from build123d import *

# Parameters (mm, degrees)
EXTRUDE_3_DEPTH = 1.169927
EXTRUDE_4_DEPTH = 5
EXTRUDE_5_DEPTH = 5


with BuildPart() as part:
    # 草图2 → 凸台-拉伸3 (new body)
    with BuildSketch(Plane(origin=(0, 15, 0), x_dir=(1, 0, 0), z_dir=(0, 1, 0))):
        with BuildLine():
            Line((-24.853345035, 10.461479878), (-24.853345035, 0.41148))
            Line((-24.853345035, 0.41148), (-2.753344966, 0.41148))
            Line((-2.753344966, 0.41148), (-2.753344966, 10.461479878))
            Line((-2.753344966, 10.461479878), (0.013999939, 10.461479878))
            ThreePointArc((0.013999939, 10.461479878), (3.195980454, 9.143460393), (4.513999939, 5.961479878))
            Line((4.513999939, 5.961479878), (4.513999939, -14.938520122))
            ThreePointArc((4.513999939, -14.938520122), (3.195980454, -18.120500638), (0.013999939, -19.438520122))
            Line((0.013999939, -19.438520122), (-27.986000061, -19.438520122))
            ThreePointArc((-27.986000061, -19.438520122), (-31.167980576, -18.120500638), (-32.486000061, -14.938520122))
            Line((-32.486000061, -14.938520122), (-32.486000061, 5.961479878))
            ThreePointArc((-32.486000061, 5.961479878), (-31.167980576, 9.143460393), (-27.986000061, 10.461479878))
            Line((-27.986000061, 10.461479878), (-24.853345035, 10.461479878))
        make_face()
    extrude(amount=EXTRUDE_3_DEPTH)

    # 草图4 → 凸台-拉伸4 (add)
    with BuildSketch(Plane.XZ.offset(-15)):
        with BuildLine():
            Line((-23.193000031, 0.4), (-28.386000061, 0.4))
            Line((-28.386000061, 0.4), (-28.386000061, -0.81148))
            Line((-28.386000061, -0.81148), (-24.853345035, -0.81148))
            Line((-24.853345035, -0.81148), (-24.853345035, -10.461479878))
            Line((-24.853345035, -10.461479878), (-27.986000061, -10.461479878))
            ThreePointArc((-27.986000061, -10.461479878), (-31.167980576, -9.143460393), (-32.486000061, -5.961479878))
            Line((-32.486000061, -5.961479878), (-32.486000061, 14.938520122))
            ThreePointArc((-32.486000061, 14.938520122), (-31.167980576, 18.120500638), (-27.986000061, 19.438520122))
            Line((-27.986000061, 19.438520122), (0.013999939, 19.438520122))
            ThreePointArc((0.013999939, 19.438520122), (3.195980454, 18.120500638), (4.513999939, 14.938520122))
            Line((4.513999939, 14.938520122), (4.513999939, -5.961479878))
            ThreePointArc((4.513999939, -5.961479878), (3.195980454, -9.143460393), (0.013999939, -10.461479878))
            Line((0.013999939, -10.461479878), (-2.753344966, -10.461479878))
            Line((-2.753344966, -10.461479878), (-2.753344966, -0.81148))
            Line((-2.753344966, -0.81148), (0.4, -0.81148))
            Line((0.4, -0.81148), (0.4, 0.4))
            Line((0.4, 0.4), (-5.193000031, 0.4))
            Line((-5.193000031, 0.4), (-5.193000031, 3.4))
            Line((-5.193000031, 3.4), (-23.193000031, 3.4))
            Line((-23.193000031, 3.4), (-23.193000031, 0.4))
        make_face()
    extrude(amount=EXTRUDE_4_DEPTH)

    # 草图5 → 凸台-拉伸5 (add)
    with BuildSketch(Plane.XZ.offset(-10)):
        with BuildLine():
            Line((-2.753344966, -8.561479878), (0.013999939, -8.561479878))
            ThreePointArc((0.013999939, -8.561479878), (1.85247757, -7.799957509), (2.613999939, -5.961479878))
            Line((2.613999939, -5.961479878), (2.613999939, 14.938520122))
            ThreePointArc((2.613999939, 14.938520122), (1.85247757, 16.776997753), (0.013999939, 17.538520122))
            Line((0.013999939, 17.538520122), (-27.986000061, 17.538520122))
            ThreePointArc((-27.986000061, 17.538520122), (-29.824477692, 16.776997753), (-30.586000061, 14.938520122))
            Line((-30.586000061, 14.938520122), (-30.586000061, -5.961479878))
            ThreePointArc((-30.586000061, -5.961479878), (-29.824477692, -7.799957509), (-27.986000061, -8.561479878))
            Line((-27.986000061, -8.561479878), (-24.768224203, -8.561479878))
            Line((-24.768224203, -8.561479878), (-24.768224203, -7.061479878))
            Line((-24.768224203, -7.061479878), (-27.986000061, -7.061479878))
            ThreePointArc((-27.986000061, -7.061479878), (-28.76381752, -6.739297337), (-29.086000061, -5.961479878))
            Line((-29.086000061, -5.961479878), (-29.086000061, 14.938520122))
            ThreePointArc((-29.086000061, 14.938520122), (-28.76381752, 15.716337581), (-27.986000061, 16.038520122))
            Line((-27.986000061, 16.038520122), (0.013999939, 16.038520122))
            ThreePointArc((0.013999939, 16.038520122), (0.791817398, 15.716337581), (1.113999939, 14.938520122))
            Line((1.113999939, 14.938520122), (1.113999939, -5.961479878))
            ThreePointArc((1.113999939, -5.961479878), (0.791817398, -6.739297337), (0.013999939, -7.061479878))
            Line((0.013999939, -7.061479878), (-2.753344966, -7.061479878))
            Line((-2.753344966, -7.061479878), (-2.753344966, -8.561479878))
        make_face()
    extrude(amount=EXTRUDE_5_DEPTH)


solid = part.part
Work out the finished part from the listing and answer in its coordinate system (mm). A direction names the side the tool comes from. Give positions to 0.01 mm unless a question says otherwise; leave off trailing zeros. Write each loop counter-clockwise with the first axis right and the second up, starting at its lowest first coordinate (ties: lowest second). Pieces come first, ordered by that corner, then holes. Notation, with made-up numbers: (-4, -34.75) - (25, -34.75) arc R35 cw to (25, 0.25) - close; hole circle Ø2 at (29, 81.5). An arc over 180 degrees is marked (long way). One line per item, written item: value. Start each with the question number.
1. Given pin 1 (4 mm diameter, centred on x = -12.5, y = 7, fed in from -Z); pin 2 (3 mm diameter, centred on y = 8, z = 1, fed in from -X); pin 3 (7 mm diameter, centred on x = -18.5, z = 1.5, fed in from -Y), each flat-ended and moving along its own axis, determine where each tip first touches the part or whether it passes through.
2. Find section B-B (x = -16.5). Write down the section's boundary in (y, z).
3. Consider probe 1 along X at (y, z) = (12.75, 2); probe 2 along Z at (x, y) = (-26.5, 10.5); probe 3 along X at (y, z) = (7.75, 12.5). Determine where each line is inside the solid, lowest interval first.
4. For a pull along Z with two mould halves and no side action, classify faces 1 (the flat face through (-5.193, 13, 2)), 2 (the cylindrical face through (-29.845, 7.535, -7.78)), 3 (the flat face through (-2, 13, 0.4)) as +Z half, -Z half, draft (parallel to the pull), parting line (faces both ways), or undercut.
5. Find section A-A (z = -1.5). Write down the section's boundary in (x, y).
6. For faces 4 (the cylindrical face through (1.83, 7.54, -7.82)), 5 (the cylindrical face through (0.783, 7.535, 15.725)), 6 (the flat face through (-14, 8, 17.539)), determine the directions among +Z, -Z, +X, -X, +Y, -Y from which every point of the face is accessible in a straight line to the end or side of a thin tool.
7. Find section C-C (z = 10.5). Write down the section's boundary in (x, y), then the cut area to 3 significant figures.
8. Find section D-D (y = 6.5). Write down the section's boundary in (x, z), then the cut area to 3 significant figures.
Geometry results:
1. pin 1: z = 16.04
1. pin 2: x = -30.59
1. pin 3: y = 10
2. outline: (5, 16.04) - (10, 16.04) - (10, 3.4) - (15, 3.4) - (15, -0.41) - (16.17, -0.41) - (16.17, 19.44) - (10, 19.44) - (10, 17.54) - (5, 17.54) - close
3. probe 1: -32.49 to -23.19, -5.19 to 4.51
3. probe 2: -10.46 to -0.81, 0.4 to 19.44
3. probe 3: -30.59 to -29.09, 1.11 to 2.61
4. face 1: draft
4. face 2: -Z half
4. face 3: undercut
5. outline: (-32.49, 10) - (-30.59, 10) - (-30.59, 5) - (-29.09, 5) - (-29.09, 10) - (-24.85, 10) - (-24.85, 16.17) - (-32.49, 16.17) - close; (-2.75, 10) - (1.11, 10) - (1.11, 5) - (2.61, 5) - (2.61, 10) - (4.51, 10) - (4.51, 16.17) - (-2.75, 16.17) - close
6. face 4: -Z, +X, -Y
6. face 5: -Y
6. face 6: +Z, +X, -X, -Y
7. outline: (-32.49, 10) - (-30.59, 10) - (-30.59, 5) - (-29.09, 5) - (-29.09, 10) - (1.11, 10) - (1.11, 5) - (2.61, 5) - (2.61, 10) - (4.51, 10) - (4.51, 16.17) - (-32.49, 16.17) - close
7. area: 243 mm2
8. outline: (-30.59, -5.96) arc R2.6 ccw to (-27.99, -8.56) - (-24.77, -8.56) - (-24.77, -7.06) - (-27.99, -7.06) arc R1.1 cw to (-29.09, -5.96) - (-29.09, 14.94) arc R1.1 cw to (-27.99, 16.04) - (0.01, 16.04) arc R1.1 cw to (1.11, 14.94) - (1.11, -5.96) arc R1.1 cw to (0.01, -7.06) - (-2.75, -7.06) - (-2.75, -8.56) - (0.01, -8.56) arc R2.6 ccw to (2.61, -5.96) - (2.61, 14.94) arc R2.6 ccw to (0.01, 17.54) - (-27.99, 17.54) arc R2.6 ccw to (-30.59, 14.94) - close
8. area: 131 mm2
